```python
from build123d import *

# Parameters (mm, degrees)
F0_W      = 152.4
F0_H      = 152.4
F1_DEPTH  = 6.35
F2_W      = 38.1
F2_H      = 6.35
F3_DEPTH  = 25.4
F4_W      = 6.35
F4_H      = 38.1
F5_DEPTH  = 25.4
F6_W      = 38.1
F6_H      = 6.35
F7_DEPTH  = 25.4
F8_W      = 6.35
F8_H      = 38.1
F9_DEPTH  = 25.4
F10_R     = 5.08
F11_DEPTH = 10.16
F12_R     = 3.175
F13_DEPTH = 8.89


with BuildPart() as f1:
    # F0 (on Top) → F1 (new body)
    with BuildSketch(Plane.XY):
        Rectangle(F0_W, F0_H)
    extrude(amount=F1_DEPTH)

    # F2 (on face) → F3 (cut)
    with BuildSketch(Plane.XY.offset(6.35)):
        with Locations((50.8, 0)):
            Rectangle(F2_W, F2_H)
    extrude(amount=-F3_DEPTH, mode=Mode.SUBTRACT)

    # F4 (on face) → F5 (cut)
    with BuildSketch(Plane.XY.offset(6.35)):
        with Locations((0, -50.8)):
            Rectangle(F4_W, F4_H)
    extrude(amount=-F5_DEPTH, mode=Mode.SUBTRACT)

    # F6 (on face) → F7 (cut)
    with BuildSketch(Plane.XY.offset(6.35)):
        with Locations((-50.8, 0)):
            Rectangle(F6_W, F6_H)
    extrude(amount=-F7_DEPTH, mode=Mode.SUBTRACT)

    # F8 (on face) → F9 (cut)
    with BuildSketch(Plane.XY.offset(6.35)):
        with Locations((0, 50.8)):
            Rectangle(F8_W, F8_H)
    extrude(amount=-F9_DEPTH, mode=Mode.SUBTRACT)

    # F10 (on face) → F11 (join)
    with BuildSketch(Plane.XY.offset(6.35)):
        Circle(F10_R)
    extrude(amount=F11_DEPTH)

    # F12 (on face) → F13 (cut)
    with BuildSketch(Plane.XY.offset(16.51)):
        Circle(F12_R)
    extrude(amount=-F13_DEPTH, mode=Mode.SUBTRACT)


solid = f1.part
```
Can you work these out from the model? Positions are in its coordinate system, mm. A direction names the side the tool comes from. Round coordinates to 2 decimals unless told otherwise and drop trailing zeros. Loops run counter-clockwise (first coordinate to the right, second up) from the corner with the lowest first, then second, coordinate; pieces in that order, holes last. Notation, with made-up numbers: (-11.5, -4) -> (9.5, -4) arc R15 cw to (9.5, 11) -> close; hole circle Ø7 at (16, 27.5). An arc over 180 degrees is marked (long way). Answer in a Markdown table with one row per item.
Item 1: On a 3-axis mill with a long thin cutter (end or side, diameter ignored), from which of +Z, -Z, +X, -X, +Y, -Y can I reach the whole of each face in a straight line? I mean faces 1 (the flat face through (69.85, 0, 3)), 2 (the cylindrical face through (-0.661, 5.037, 11.359)), 3 (the flat face through (-1, 76.2, 3)). Say none if no direction works.
Answer block:
| item | result |
|---|---|
| face 1 | +Z, -Z |
| face 2 | +Z |
| face 3 | +Z, -Z, +X, -X, +Y |
Item 2: We'd pull the mould along X, two halves only. Please class faces 4 (the flat face through (16, 1, 6.35)), 5 (the flat face through (76.2, -1, 3)), 6 (the flat face through (-31.75, 0, 3)), 7 (the flat face through (-76.2, -1, 3)): released by +X, released by -X, zero draft, split by the parting line, or undercut.
Answer block:
| item | result |
|---|---|
| face 4 | zero draft |
| face 5 | released by +X |
| face 6 | undercut |
| face 7 | released by -X |
Item 3: Suppose I cut it at B-B, the plane x = -56.5. List the corners of the cut face in (y, z) for me (3 decimals).
Answer block:
| item | result |
|---|---|
| outline | (-76.2, 0) -> (-3.175, 0) -> (-3.175, 6.35) -> (-76.2, 6.35) -> close; (3.175, 0) -> (76.2, 0) -> (76.2, 6.35) -> (3.175, 6.35) -> close |
Item 4: If I drill on probe 1 along Y at (x, z) = (0, 12.25) (3 decimals); probe 2 along X at (y, z) = (-50.5, 1.5) (3 decimals), over which ranges is the centre line in solid material (lowest first)?
Answer block:
| item | result |
|---|---|
| probe 1 | -5.08 to -3.175, 3.175 to 5.08 |
| probe 2 | -76.2 to -3.175, 3.175 to 76.2 |
Item 5: Suppose I cut it at A-A, the plane y = 0. List the corners of the cut face in (x, z) for me (3 decimals), plus the area to 3 significant figures.
Answer block:
| item | result |
|---|---|
| outline | (-76.2, 0) -> (-69.85, 0) -> (-69.85, 6.35) -> (-76.2, 6.35) -> close; (-31.75, 0) -> (31.75, 0) -> (31.75, 6.35) -> (5.08, 6.35) -> (5.08, 16.51) -> (3.175, 16.51) -> (3.175, 7.62) -> (-3.175, 7.62) -> (-3.175, 16.51) -> (-5.08, 16.51) -> (-5.08, 6.35) -> (-31.75, 6.35) -> close; (69.85, 0) -> (76.2, 0) -> (76.2, 6.35) -> (69.85, 6.35) -> close |
| area | 531 mm² |
Item 6: Will these pins go through, and if not, where does the flat tip stop? P1, Ø3, axis at x = 0.5, y = 0, coming from the +Z side; P2, Ø2, axis at x = -31, y = 52.5, coming from the +Z side.
Answer block:
| item | result |
|---|---|
| P1 | z = 7.62 |
| P2 | z = 6.35 |
